from build123d import *

# Parameters (mm, degrees)
SKETCH1_W           = 47.09116882
SKETCH1_H           = 77.09116882
BOSS_EXTRUDE1_DEPTH = 1.5
SKETCH2_W           = 47.09116882
SKETCH2_H           = 77.09116882
SKETCH2_W_2         = 44.545584412
SKETCH2_H_2         = 74.545584412
BOSS_EXTRUDE2_DEPTH = 20
FILLET4_R           = 1
SKETCH9_W           = 8.4
SKETCH9_H           = 2.6
CUT_EXTRUDE4_DEPTH  = 2
FILLET5_R           = 1
SKETCH10_W          = 2.5
SKETCH10_H          = 19.895622202
SKETCH10_W_2        = 15
SKETCH10_H_2        = 2.746977623
BOSS_EXTRUDE4_DEPTH = 5
SKETCH11_W          = 14
SKETCH11_H          = 4
CUT_EXTRUDE5_DEPTH  = 10
SKETCH12_W          = 75.09116882
SKETCH12_H          = 3
BOSS_EXTRUDE5_DEPTH = 46
SKETCH13_W          = 41.13137085
SKETCH13_H          = 71.13137085
CUT_EXTRUDE6_DEPTH  = 3
FILLET6_R           = 1
CUT_EXTRUDE8_DEPTH  = 3


with BuildPart() as part:
    # Sketch1 → Boss-Extrude1 (new body)
    with BuildSketch(Plane(origin=(0, 0, 0), x_dir=(1, 0, 0), z_dir=(0, 1, 0))):
        with Locations((23.54558441, -38.54558441)):
            Rectangle(SKETCH1_W, SKETCH1_H)
    extrude(amount=BOSS_EXTRUDE1_DEPTH)

    # Sketch2 → Boss-Extrude2 (add)
    with BuildSketch(Plane(origin=(0, 1.5, 0), x_dir=(1, 0, 0), z_dir=(0, 1, 0))):
        with Locations((23.54558441, -38.54558441)):
            Rectangle(SKETCH2_W, SKETCH2_H)
        with Locations((23.545584412, -38.545584412)):
            Rectangle(SKETCH2_W_2, SKETCH2_H_2, mode=Mode.SUBTRACT)
    extrude(amount=BOSS_EXTRUDE2_DEPTH)

    # Fillet4
    fillet4_edges = [part.edges().sort_by_distance(p)[0] for p in [
        (1.272792206, 11.5, 75.818376618),
        (45.818376618, 11.5, 75.818376618),
        (45.818376618, 11.5, 1.272792206),
        (1.272792206, 11.5, 1.272792206),
        (0, 10.75, 0),
        (47.09116882, 10.75, 0),
        (47.09116882, 10.75, 77.09116882),
        (0, 10.75, 77.09116882),
    ]]
    fillet(fillet4_edges, radius=FILLET4_R)

    # Sketch9 → Cut-Extrude4 (cut)
    with BuildSketch(Plane(origin=(47.09116882, 0, 0), x_dir=(0, 0, -1), z_dir=(1, 0, 0))):
        with Locations((-6.471655529, 15.764642051)):
            Rectangle(SKETCH9_W, SKETCH9_H)
    extrude(amount=-CUT_EXTRUDE4_DEPTH, mode=Mode.SUBTRACT)

    # Fillet5
    # the kernel refuses this fillet: 1 mm, written as the material it adds along each edge
    with BuildSketch(Plane(origin=(47.09116882, 17.064642051, 10.671655529), x_dir=(0, 0, -1), z_dir=(-1, 0, 0))) as fillet5_piece_1:
        with BuildLine():
            CenterArc((FILLET5_R, FILLET5_R), FILLET5_R, 180, 90)
            Line((0, FILLET5_R), (0, 0))
            Line((0, 0), (FILLET5_R, 0))
        make_face()
    extrude(amount=1.272792202)
    with BuildSketch(Plane(origin=(47.09116882, 14.464642051, 2.271655529), x_dir=(0, 0, 1), z_dir=(-1, 0, 0))) as fillet5_piece_2_section:
        with BuildLine():
            CenterArc((FILLET5_R, FILLET5_R), FILLET5_R, 180, 90)
            Line((0, FILLET5_R), (0, 0))
            Line((0, 0), (FILLET5_R, 0))
        make_face()
    fillet5_piece_2 = extrude(amount=3.772792848, mode=Mode.PRIVATE)
    fillet5_piece_2 = split(fillet5_piece_2, bisect_by=Plane(origin=(45.818376618, 14.688009946, 2.495023498), z_dir=(1, 0, 0)), keep=Keep.TOP, mode=Mode.PRIVATE)
    add(fillet5_piece_2)
    with BuildSketch(Plane(origin=(47.09116882, 17.064642051, 2.271655529), x_dir=(0, -1, 0), z_dir=(-1, 0, 0))) as fillet5_piece_3_section:
        with BuildLine():
            CenterArc((FILLET5_R, FILLET5_R), FILLET5_R, 180, 90)
            Line((0, FILLET5_R), (0, 0))
            Line((0, 0), (FILLET5_R, 0))
        make_face()
    fillet5_piece_3 = extrude(amount=3.772792848, mode=Mode.PRIVATE)
    fillet5_piece_3 = split(fillet5_piece_3, bisect_by=Plane(origin=(45.818376618, 16.841274155, 2.495023498), z_dir=(1, 0, 0)), keep=Keep.TOP, mode=Mode.PRIVATE)
    add(fillet5_piece_3)
    with BuildSketch(Plane(origin=(47.09116882, 14.464642051, 10.671655529), x_dir=(0, 0, -1), z_dir=(-1, 0, 0))) as fillet5_piece_4:
        with BuildLine():
            CenterArc((FILLET5_R, -FILLET5_R), FILLET5_R, 90, 90)
            Line((0, -FILLET5_R), (0, 0))
            Line((0, 0), (FILLET5_R, 0))
        make_face()
    extrude(amount=1.272792202)

    # Sketch10 → Boss-Extrude4 (add)
    with BuildSketch(Plane(origin=(0, 1.5, 0), x_dir=(1, 0, 0), z_dir=(0, 1, 0))):
        with Locations((2.082813384, -63.025844565)):
            Rectangle(SKETCH10_W, SKETCH10_H)
        with Locations((7.824900782, -24.444887807)):
            Rectangle(SKETCH10_W_2, SKETCH10_H_2)
        with Locations((39.244805213, -24.444887807)):
            Rectangle(SKETCH10_W_2, SKETCH10_H_2)
        with Locations((2.082813384, -38.610908672)):
            Rectangle(SKETCH10_W, SKETCH10_H)
        with Locations((45.295584412, -38.610908672)):
            Rectangle(SKETCH10_W, SKETCH10_H)
        with Locations((45.295584412, -63.025844565)):
            Rectangle(SKETCH10_W, SKETCH10_H)
    extrude(amount=BOSS_EXTRUDE4_DEPTH)

    # Sketch11 → Cut-Extrude5 (cut)
    with BuildSketch(Plane.XY.offset(77.09116882)):
        with Locations((23.545584412, 17.117945241)):
            Rectangle(SKETCH11_W, SKETCH11_H)
    extrude(amount=-CUT_EXTRUDE5_DEPTH, mode=Mode.SUBTRACT)

    # Sketch12 → Boss-Extrude5 (add)
    with BuildSketch(Plane(origin=(47.09116882, 0, 0), x_dir=(0, 0, -1), z_dir=(1, 0, 0))):
        with Locations((-38.54558441, 12)):
            Rectangle(SKETCH12_W, SKETCH12_H)
    extrude(amount=-BOSS_EXTRUDE5_DEPTH)

    # Sketch13 → Cut-Extrude6 (cut)
    with BuildSketch(Plane(origin=(0, 13.5, 0), x_dir=(1, 0, 0), z_dir=(0, 1, 0))):
        with Locations((23.545584412, -38.545584412)):
            Rectangle(SKETCH13_W, SKETCH13_H)
    extrude(amount=-CUT_EXTRUDE6_DEPTH, mode=Mode.SUBTRACT)

    # Fillet6
    fillet6_edges = [part.edges().sort_by_distance(p)[0] for p in [
        (44.111269837, 12, 74.111269837),
        (2.979898987, 12, 74.111269837),
        (2.979898987, 12, 2.979898987),
        (44.111269837, 12, 2.979898987),
    ]]
    fillet(fillet6_edges, radius=FILLET6_R)

    # Sketch14 → Cut-Extrude8 (cut)
    with BuildSketch(Plane(origin=(0, 13.5, 0), x_dir=(1, 0, 0), z_dir=(0, 1, 0))):
        with BuildLine():
            Line((1.272792206, -11.492184631), (12.679197534, -11.492184631))
            Line((12.679197534, -11.492184631), (12.679197534, -1.272792206))
            Line((12.679197534, -1.272792206), (2.272792206, -1.272792206))
            ThreePointArc((2.272792206, -1.272792206), (1.565685425, -1.565685425), (1.272792206, -2.272792206))
            Line((1.272792206, -2.272792206), (1.272792206, -11.492184631))
        make_face()
    extrude(amount=-CUT_EXTRUDE8_DEPTH, mode=Mode.SUBTRACT)


solid = part.part
The model under review builds one solid part; all positions refer to its coordinate system, in mm. A direction names the side the tool comes from. Round coordinates to 2 decimals unless told otherwise and drop trailing zeros. Write each loop counter-clockwise with the first axis right and the second up, starting at its lowest first coordinate (ties: lowest second). Pieces come first, ordered by that corner, then holes. Notation, with made-up numbers: (52.25, -22) -> (79.25, -22) arc R20 ccw to (79.25, -8) -> close; hole circle Ø2 at (-27, 82). An arc over 180 degrees is marked (long way). Answer as a JSON object with one key per item and string values.
1. Machinability: for faces 3 (the face through (45, 6.5, 63)), 4 (the face through (12.679, 12, 2)), which of the approach directions +Z, -Z, +X, -X, +Y, -Y give a long, thin tool a straight path to every point of the face, cutting with its end or side? Answer none if there is none.
Results found:
{"face 3": "none", "face 4": "+Y"}
2. To check wall thickness, follow line 1 along X through (y, z) = (11, 41.5); line 2 along Z through (x, y) = (15, 4.25); line 3 along Z through (x, y) = (27, 12). State the ranges of each line that lie inside material, in increasing order.
Results found:
{"line 1": "x = 0 to 2.98, 44.11 to 47.09", "line 2": "z = 0 to 1.27, 23.07 to 25.82, 75.82 to 77.09", "line 3": "z = 0 to 2.98, 74.11 to 77.09"}
3. We need section B-B on z = 5. State the section outline as (x, y) points.
Results found:
{"outline": "(0, 0) -> (47.09, 0) -> (47.09, 14.46) -> (45.82, 14.46) -> (45.82, 13.5) -> (44.11, 13.5) -> (44.11, 10.5) -> (45.82, 10.5) -> (45.82, 1.5) -> (1.27, 1.5) -> (1.27, 21.5) -> (0, 21.5) -> close; (45.82, 17.06) -> (47.09, 17.06) -> (47.09, 21.5) -> (45.82, 21.5) -> close"}
4. Clearance check with a flat-ended pin moving along its axis: pin 1 (0.5 mm diameter, centred on x = 44.5, z = 42.5, fed in from +Y). State where the tip first meets the part, or that it passes through.
Results found:
{"pin 1": "stops at y = 13.5"}
5. We need section A-A on x = 21. State the section outline as (y, z) points, and give its area (3 significant figures).
Results found:
{"outline": "(0, 0) -> (21.5, 0) -> (21.5, 1.27) -> (13.5, 1.27) -> (13.5, 2.98) -> (10.5, 2.98) -> (10.5, 1.27) -> (1.5, 1.27) -> (1.5, 75.82) -> (10.5, 75.82) -> (10.5, 74.11) -> (13.5, 74.11) -> (13.5, 75.82) -> (15.12, 75.82) -> (15.12, 77.09) -> (0, 77.09) -> close; (19.12, 75.82) -> (21.5, 75.82) -> (21.5, 77.09) -> (19.12, 77.09) -> close", "area": "172 mm^2"}
6. We need section D-D on x = 6. State the section outline as (y, z) points.
Results found:
{"outline": "(0, 0) -> (21.5, 0) -> (21.5, 1.27) -> (1.5, 1.27) -> (1.5, 23.07) -> (6.5, 23.07) -> (6.5, 25.82) -> (1.5, 25.82) -> (1.5, 75.82) -> (10.5, 75.82) -> (10.5, 74.11) -> (13.5, 74.11) -> (13.5, 75.82) -> (21.5, 75.82) -> (21.5, 77.09) -> (0, 77.09) -> close"}
7. We need section C-C on y = 12.5. State the section outline as (x, z) points.
Results found:
{"outline": "(0, 1) arc R1 ccw to (1, 0) -> (46.09, 0) arc R1 ccw to (47.09, 1) -> (47.09, 76.09) arc R1 ccw to (46.09, 77.09) -> (1, 77.09) arc R1 ccw to (0, 76.09) -> close; hole (1.27, 2.27) arc R1 ccw to (2.27, 1.27) -> (12.68, 1.27) -> (12.68, 2.98) -> (43.11, 2.98) arc R1 ccw to (44.11, 3.98) -> (44.11, 73.11) arc R1 ccw to (43.11, 74.11) -> (3.98, 74.11) arc R1 ccw to (2.98, 73.11) -> (2.98, 11.49) -> (1.27, 11.49) -> close"}
8. The part is to be moulded in two halves that separate along Y. For faces 1 (the face through (23, 9, 1.273)), 2 (the face through (0, 11, 39)), say which applies: pulls with the +Y half, pulls with the -Y half, needs draft (parallel to the pull), parting line crosses it, or undercut.
Results found:
{"face 1": "undercut", "face 2": "needs draft"}
